```python
from build123d import *

# Parameters (mm, degrees)
SKETCH030_R     = 35.5
PAD012_DEPTH    = 30
SKETCH031_R     = 24
POCKET_DEPTH    = 25
SKETCH032_R     = 8
PAD013_DEPTH    = 12
POCKET001_DEPTH = 3
SKETCH004_R     = 1.5
POCKET002_DEPTH = 3
FILLET016_R     = 3
FILLET017_R     = 3


with BuildPart() as part:
    # Sketch030 → Pad012 (new body)
    with BuildSketch(Plane.YZ):
        with Locations((-2.086398, 2.086246)):
            Circle(SKETCH030_R)
    extrude(amount=PAD012_DEPTH)

    # Sketch031 (on Face2 of Pad012) → Pocket (cut)
    with BuildSketch(Plane(origin=(0, 0, 0), x_dir=(0, 1, 0), z_dir=(-1, 0, 0))):
        with Locations((-1.664763, -2.119737)):
            Circle(SKETCH031_R)
    extrude(amount=-POCKET_DEPTH, mode=Mode.SUBTRACT)

    # Sketch032 (on Face5 of Pocket) → Pad013 (join)
    with BuildSketch(Plane(origin=(25, 0, 0), x_dir=(0, 1, 0), z_dir=(-1, 0, 0))):
        with Locations((-1.350817, -2.732668)):
            Circle(SKETCH032_R)
    extrude(amount=PAD013_DEPTH)

    # Sketch033 (on Face7 of Pad013) → Pocket001 (cut)
    with BuildSketch(Plane(origin=(13, 0, 0), x_dir=(0, 1, 0), z_dir=(-1, 0, 0))):
        Polygon((-1.111872, 4.248012), (-7.222761, 0.700721), (-7.206161, -6.365109), (-1.078672, -9.883648), (5.032216, -6.336357), (5.015616, 0.729474), align=None)
    extrude(amount=-POCKET001_DEPTH, mode=Mode.SUBTRACT)

    # Sketch004 (on Face14 of Pocket001) → Pocket002 (cut)
    with BuildSketch(Plane(origin=(16, 0, 0), x_dir=(0, 1, 0), z_dir=(-1, 0, 0))):
        with Locations((-0.927213, -2.793039)):
            Circle(SKETCH004_R)
    extrude(amount=-POCKET002_DEPTH, mode=Mode.SUBTRACT)

    # Fillet016
    fillet016_edges = [part.edges().sort_by_distance(p)[0] for p in [
        (0, -37.586398, 2.086246),
    ]]
    fillet(fillet016_edges, radius=FILLET016_R)

    # Fillet017
    fillet017_edges = [part.edges().sort_by_distance(p)[0] for p in [
        (30, -37.586398, 2.086246),
    ]]
    fillet(fillet017_edges, radius=FILLET017_R)


with BuildPart() as part_1:
    # Body001 placement: moved
    add(part.part.moved(Location((77, -11, 5))))


solid = part_1.part
```
The model under review builds one solid part; all positions refer to its coordinate system, in mm. A direction names the side the tool comes from. Coordinates: 2 decimals unless noted, no trailing zeros. Loops run counter-clockwise (first coordinate to the right, second up) from the corner with the lowest first, then second, coordinate; pieces in that order, holes last. Notation, with made-up numbers: (83, -19.75) -> (88, -19.75) arc R14 ccw to (88, 1.25) -> close; hole circle Ø2 at (47.5, 56). An arc over 180 degrees is marked (long way). Answer as CSV lines item,"result".
Item 1: Machinability: for faces 4 (the flat face through (102, -18, 1)), 5 (the flat face through (77, -30, -10)), which of the approach directions +Z, -Z, +X, -X, +Y, -Y give a long, thin tool a straight path to every point of the face, cutting with its end or side? Answer none if there is none.
Results below:
face 4,"-X"
face 5,"+Z, -Z, -X, +Y, -Y"
Item 2: Take a section at B-B, the plane x = 101. State the section outline as (y, z) points.
Results below:
outline,"circle Ø71 at (-13.09, 7.09); circle Ø16 at (-12.35, 7.73); hole circle Ø48 at (-12.66, 7.12)"
Item 3: Draft analysis for pull direction Z (two halves, no side actions). For faces 1 (the flat face through (90, -15, 14)), 2 (the cylindrical face through (91.832, 20.774, 17.749)), 3 (the flat face through (107, -14, 8)), state which applies: +Z half, -Z half, draft (parallel to the pull), parting line (faces both ways), or undercut.
Results below:
face 1,"undercut"
face 2,"parting line"
face 3,"draft"
Item 4: Take a section at A-A, the plane x = 95. State the section outline as (y, z) points, and give its area (3 significant figures).
Results below:
outline,"circle Ø71 at (-13.09, 7.09); circle Ø16 at (-12.35, 7.73); hole circle Ø48 at (-12.66, 7.12); hole circle Ø3 at (-11.93, 7.79)"
area,"2,340 mm2"
Item 5: Take a section at C-C, the plane x = 105. State the section outline as (y, z) points.
Results below:
outline,"circle Ø70.66 at (-13.09, 7.09)"
Item 6: Insertion check: pin 1 (2.5 mm diameter, centred on y = -11.5, z = 7, fed in from -X); pin 2 (13 mm diameter, centred on y = -9.5, z = 6, fed in from -X); pin 3 (12 mm diameter, centred on x = 84.5, y = -22, fed in from +Z). Each pin has a flat end and moves straight along its axis. Give the tip position at first contact, or say it passes through.
Results below:
pin 1,"stops at x = 93"
pin 2,"stops at x = 90"
pin 3,"stops at z = 42.47"
Item 7: For L1, parallel to Z at x = 87, y = -12; L2, parallel to Z at x = 92, y = -12.5; L3, parallel to Z at x = 90, y = 1.5, list the stretches that pass through material, from the lowest coordinate up.
Results below:
L1,"z = -28.4 to -16.87, 31.11 to 42.57"
L2,"z = -28.41 to -16.88, -0.27 to 0.98, 14.64 to 15.73, 31.12 to 42.58"
L3,"z = -25.28 to -12.25, 26.49 to 39.45"
